```python
from build123d import *

# Parameters (mm, degrees)
SKETCH2_W               = 1
SKETCH2_H               = 80
CUT_EXTRUDE1_DEPTH      = 81.199750623
CUT_EXTRUDE1_DEPTH_BACK = 81.199750623
SKETCH3_R               = 1.25


with BuildPart() as part:
    # Sketch2 → revolve 1 (revolve)
    with BuildSketch(Plane(origin=(0, 0, 0), x_dir=(0, 0, -1), z_dir=(1, 0, 0))):
        with Locations((3.5, 40)):
            Rectangle(SKETCH2_W, SKETCH2_H)
    revolve(axis=Axis((0, 0, 0), (0, 1, 0)))

    # Sketch3 → Cut-Extrude1 (cut, two sides: drawn at the far end of the back side and taken through both)
    with BuildSketch(Plane(origin=(0, 0, 0), x_dir=(0, 0, -1), z_dir=(1, 0, 0)).offset(-CUT_EXTRUDE1_DEPTH_BACK)):
        with Locations(Location((0, 5, 0), (0, 0, 180))):
            Circle(SKETCH3_R)
        with Locations(Location((0, 70, 0), (0, 0, 180))):
            Circle(SKETCH3_R)
    extrude(amount=CUT_EXTRUDE1_DEPTH + CUT_EXTRUDE1_DEPTH_BACK, mode=Mode.SUBTRACT)


solid = part.part
```
Design review of the part built by this model. Coordinates are the model's own, in mm. Give positions to 0.01 mm unless a question says otherwise; leave off trailing zeros. Write each loop counter-clockwise with the first axis right and the second up, starting at its lowest first coordinate (ties: lowest second). Pieces come first, ordered by that corner, then holes. Notation, with made-up numbers: (-36.5, 14) - (-31.5, 14) arc R36 ccw to (-31.5, 50) - close; hole circle Ø8 at (50.5, -36). An arc over 180 degrees is marked (long way). Return JSON: item names as keys, results as strings. Group by question number.
(1) We need section A-A, the plane x = 1.25. Give the boundary of the cut face in (y, z).
(2) We need section B-B, the plane z = 0. Give the boundary of the cut face in (x, y).
(3) We need section C-C, the plane y = 5. Give the boundary of the cut face in (x, z).
(4) Insertion check: pin 1 (2 mm diameter, centred on y = 5, z = 0, fed in from +X); pin 2 (3 mm diameter, centred on x = -3, y = 9.5, fed in from -Z). Each pin has a flat end and moves straight along its axis. Give the tip position at first contact, or say it passes through.
(5) To check wall thickness, follow probe 1 along Y at (x, z) = (3.6, 0); probe 2 along Z at (x, y) = (0, 62); probe 3 along X at (y, z) = (60.5, -2). State the ranges of each line that lie inside material, in increasing order.
(6) Mouldability with a two-part tool opening along Z and no side actions: class faces 1 (the cylindrical face through (-3.375, 5.479, 1.155)), 2 (the cylindrical face through (-3.375, 70.479, 1.155)), 3 (the flat face through (-3, 0, 1)), 4 (the cylindrical face through (1.532, 40.56, -3.695)) as +Z half, -Z half, draft (parallel to the pull), parting line (faces both ways), or undercut.
Reported:
{
 "1": {"outline": "(0, -3.8) - (80, -3.8) - (80, -2.73) - (0, -2.73) - close; (0, 2.73) - (80, 2.73) - (80, 3.8) - (0, 3.8) - close"},
 "2": {"outline": "(-4, 0) - (-3, 0) - (-3, 3.75) - (-4, 3.75) - close; (-4, 6.25) - (-3, 6.25) - (-3, 68.75) - (-4, 68.75) - close; (-4, 71.25) - (-3, 71.25) - (-3, 80) - (-4, 80) - close; (3, 0) - (4, 0) - (4, 3.75) - (3, 3.75) - close; (3, 6.25) - (4, 6.25) - (4, 68.75) - (3, 68.75) - close; (3, 71.25) - (4, 71.25) - (4, 80) - (3, 80) - close"},
 "3": {"outline": "(-3.8, -1.25) arc R4 ccw to (3.8, -1.25) - (2.73, -1.25) arc R3 cw to (-2.73, -1.25) - close; (-3.8, 1.25) - (-2.73, 1.25) arc R3 cw to (2.73, 1.25) - (3.8, 1.25) arc R4 ccw to start"},
 "4": {"pin 1": "passes through", "pin 2": "stops at z = -3.71"},
 "5": {"probe 1": "y = 0 to 3.75, 6.25 to 68.75, 71.25 to 80", "probe 2": "z = -4 to -3, 3 to 4", "probe 3": "x = -3.46 to -2.24, 2.24 to 3.46"},
 "6": {"face 1": "undercut", "face 2": "undercut", "face 3": "draft", "face 4": "parting line"}
}
